from build123d import *

# Parameters (mm, degrees)
CROQUIS1_R              = 25
SALIENTE_EXTRUIR1_DEPTH = 10
CROQUIS2_R              = 5
SALIENTE_EXTRUIR2_DEPTH = 30


with BuildPart() as part:
    # Croquis1 → Saliente-Extruir1 (new body)
    with BuildSketch(Plane(origin=(0, 0, 0), x_dir=(1, 0, 0), z_dir=(0, 1, 0))):
        with Locations(Location((0, 0, 0), (0, 0, 270))):
            Circle(CROQUIS1_R)
    extrude(amount=SALIENTE_EXTRUIR1_DEPTH)

    # Croquis2 → Saliente-Extruir2 (add)
    with BuildSketch(Plane(origin=(0, 10, 0), x_dir=(1, 0, 0), z_dir=(0, 1, 0))):
        with Locations(Location((0, 0, 0), (0, 0, 270))):
            Circle(CROQUIS2_R)
    extrude(amount=SALIENTE_EXTRUIR2_DEPTH)

    # Croquis4 → Revolución1 (revolve)
    with BuildSketch(Plane.XY, mode=Mode.PRIVATE) as revoluci_n1_sk:
        with BuildLine():
            Line((5, 16.931653532), (5, 10))
            Line((5, 10), (25, 10))
            add(Edge.make_bspline(
                [(25, 10), (16.233689239, 16.931653532), (5, 16.931653532)],
                knots=[0, 0, 0, 1, 1, 1], degree=2))
        make_face()
    revolve(revoluci_n1_sk.sketch.rotate(Axis((0, 40, 0), (0, -1, 0)), 90), axis=Axis((0, 40, 0), (0, -1, 0)))


solid = part.part
Read the model definition and answer for the solid it produces. Units are mm, in the model's axes. A direction names the side the tool comes from. Round coordinates to 2 decimals unless told otherwise and drop trailing zeros. Write each loop counter-clockwise with the first axis right and the second up, starting at its lowest first coordinate (ties: lowest second). Pieces come first, ordered by that corner, then holes.
1. The part is cut by section A-A, the plane y = 36. Determine the outline of the cut face in (x, z), then the cut area to 3 significant figures.
2. Straight lines are drawn through the part: L1, parallel to Y at x = 4.5, z = 4; L2, parallel to X at y = 6, z = 0; L3, parallel to X at y = 6, z = -11.5. For each, find the intervals that lie inside material, in ascending order.
3. Given pin 1 Ø5 at (x, y) = (-5.5, 30) entering from +Z; pin 2 Ø12 at (y, z) = (13, -12) entering from +X; pin 3 Ø12 at (y, z) = (18.5, 12.5) entering from -X; pin 4 Ø6 at (x, y) = (9.5, 26) entering from +Z, each flat-ended and moving along its own axis, determine where each tip first touches the part or whether it passes through.
4. Which of the six approach directions +Z, -Z, +X, -X, +Y, -Y give full straight-line access (tool end or side, diameter ignored) to faces 1 (the face through (-4.88, 28.3, -1.08)), 2 (the face through (0, 40, 0))?
Values:
1. outline: circle Ø10 at (0, 0)
1. area: 78.5 mm2
2. L1: y = 0 to 16.92
2. L2: x = -25 to 25
2. L3: x = -22.2 to 22.2
3. pin 1: stops at z = 4
3. pin 2: stops at x = 24.06
3. pin 3: stops at x = -17.97
3. pin 4: passes through
4. face 1: +Y
4. face 2: +Z, -Z, +X, -X, +Y
